Can you work these out from the model? Positions are in its coordinate system, mm. A direction names the side the tool comes from. Round coordinates to 2 decimals unless told otherwise and drop trailing zeros. Order: outer loops, then holes, each group sorted by start corner. A loop starts at its lowest first (then second) coordinate and runs counter-clockwise, first axis right, second up. Notation, with made-up numbers: (87.25, 18.5) -> (118.25, 18.5) arc R24 cw to (118.25, 28.5) -> close; hole circle Ø8 at (62.25, -13). An arc over 180 degrees is marked (long way). One line per item, written item: value.
```python
from build123d import *

# Parameters (mm, degrees)
SKETCH2_W                = 10
SKETCH2_H                = 20
BOSS_EXTRUDE1_DEPTH      = 2
BOSS_EXTRUDE1_2_DEPTH    = 2
SKETCH6_R                = 1.5
CUT_EXTRUDE1_DEPTH       = 2
BOSS_EXTRUDE2_DEPTH      = 15
BOSS_EXTRUDE2_DEPTH_BACK = 5
SKETCH7_W                = 82.998753655
SKETCH7_H                = 2
SKETCH8_R                = 1.5
SKETCH8_W                = 16
SKETCH8_H                = 2.75
CUT_EXTRUDE2_DEPTH       = 15
SKETCH9_W                = 20.030400643
SKETCH9_H                = 3
SKETCH9_W_2              = 20.007179251
CUT_EXTRUDE3_DEPTH       = 15


with BuildPart() as part:
    # Sketch2 → Boss-Extrude1 (new body)
    with BuildSketch(Plane.XY):
        with Locations((7.834645669, 10)):
            Rectangle(SKETCH2_W, SKETCH2_H)
    extrude(amount=BOSS_EXTRUDE1_DEPTH)


with BuildPart() as body_2:
    # Sketch2 → Boss-Extrude1 2 (new body)
    with BuildSketch(Plane.XY):
        with Locations((80.834645669, 10)):
            Rectangle(SKETCH2_W, SKETCH2_H)
    extrude(amount=BOSS_EXTRUDE1_2_DEPTH)


with BuildPart() as cut_extrude1_tool:
    # Sketch6 → Cut-Extrude1 (new body)
    with BuildSketch(Plane(origin=(0, 0, 0), x_dir=(-1, 0, 0), z_dir=(0, 0, -1))):
        with Locations((-80.943458849, 13)):
            Circle(SKETCH6_R)
        with Locations((-7.943458849, 13)):
            Circle(SKETCH6_R)
    extrude(amount=-CUT_EXTRUDE1_DEPTH)


with BuildPart() as part_1:
    add(part.part)

    # Cut-Extrude1: cut by cut_extrude1_tool
    add(cut_extrude1_tool.part, mode=Mode.SUBTRACT)



with BuildPart() as body_2_1:
    add(body_2.part)

    # Cut-Extrude1: cut by cut_extrude1_tool
    add(cut_extrude1_tool.part, mode=Mode.SUBTRACT)


with BuildPart() as part_2:
    add(part_1.part)

    add(body_2_1.part)  # Boss-Extrude2 merges body 2
    # Sketch7 → Boss-Extrude2 (add, two sides: drawn at the far end of the back side and taken through both)
    with BuildSketch(Plane.XY.offset(2).offset(-BOSS_EXTRUDE2_DEPTH_BACK)):
        with Locations((44.334022496, -1)):
            Rectangle(SKETCH7_W, SKETCH7_H)
    extrude(amount=BOSS_EXTRUDE2_DEPTH + BOSS_EXTRUDE2_DEPTH_BACK)

    # Sketch8 → Cut-Extrude2 (cut)
    with BuildSketch(Plane.XZ.offset(2)):
        with Locations(Location((54.084645669, 5.796272293, 0), (0, 0, 270))):
            Circle(SKETCH8_R)
        with Locations(Location((34.584645669, 5.796272293, 0), (0, 0, 270))):
            Circle(SKETCH8_R)
        with Locations((44.334645669, 1.671272293)):
            Rectangle(SKETCH8_W, SKETCH8_H)
        Polygon((24.584645669, 12.752716477), (24.584645669, 3), (2.834645669, 3), (2.834645669, 17), (85.833399324, 17), (85.833399324, 3), (64.084645669, 3), (64.084645669, 12.752716477), align=None)
    extrude(amount=-CUT_EXTRUDE2_DEPTH, mode=Mode.SUBTRACT)

    # Sketch9 → Cut-Extrude3 (cut)
    with BuildSketch(Plane(origin=(0, 0, 0), x_dir=(1, 0, 0), z_dir=(0, 1, 0))):
        with Locations((12.849845991, 1.5)):
            Rectangle(SKETCH9_W, SKETCH9_H)
        with Locations((75.829809699, 1.5)):
            Rectangle(SKETCH9_W_2, SKETCH9_H)
    extrude(amount=-CUT_EXTRUDE3_DEPTH, mode=Mode.SUBTRACT)


solid = part_2.part
```
Q1. I want a section at B-B on y = 9.5. List the corners of the cut face in (x, z) for me, plus the area to 3 significant figures.
Answers below:
outline: (2.83, 0) -> (12.83, 0) -> (12.83, 2) -> (2.83, 2) -> close; (75.83, 0) -> (85.83, 0) -> (85.83, 2) -> (75.83, 2) -> close
area: 40.0 mm^2
Q2. Please list where these lines run through material, in increasing order: line 1 along X through (y, z) = (7.75, 1); line 2 along Z through (x, y) = (12, 18.25); line 3 along Y through (x, z) = (27, 3).
Answers below:
line 1: 2.83 to 12.83, 75.83 to 85.83
line 2: 0 to 2
line 3: -2 to 0
Q3. I want a section at D-D on x = 12. List the corners of the cut face in (y, z) for me, plus the area to 3 significant figures.
Answers below:
outline: (-2, 0) -> (20, 0) -> (20, 2) -> (0, 2) -> (0, 3) -> (-2, 3) -> close
area: 46.0 mm^2
Q4. I want a section at C-C on y = 13. List the corners of the cut face in (x, z) for me.
Answers below:
outline: (2.83, 0) -> (6.44, 0) -> (6.44, 2) -> (2.83, 2) -> close; (9.44, 0) -> (12.83, 0) -> (12.83, 2) -> (9.44, 2) -> close; (75.83, 0) -> (79.44, 0) -> (79.44, 2) -> (75.83, 2) -> close; (82.44, 0) -> (85.83, 0) -> (85.83, 2) -> (82.44, 2) -> close
Q5. Will these pins go through, and if not, where does the flat tip stop? pin 1 Ø0.6 at (y, z) = (-1, -1.5) entering from +X; pin 2 Ø5 at (x, z) = (54.08, 5.8) entering from -Y; pin 3 Ø2 at (x, z) = (69.5, 0) entering from +Y; pin 4 Ø0.6 at (y, z) = (-1.5, 8.5) entering from -X.
Answers below:
pin 1: x = 65.83
pin 2: y = -2
pin 3: y = 0
pin 4: x = 24.58
Q6. I want a section at A-A on x = 51. List the corners of the cut face in (y, z) for me, plus the area to 3 significant figures.
Answers below:
outline: (-2, -3) -> (0, -3) -> (0, 0.3) -> (-2, 0.3) -> close; (-2, 3.05) -> (0, 3.05) -> (0, 12.75) -> (-2, 12.75) -> close
area: 26.0 mm^2
Q7. We'd pull the mould along X, two halves only. Please class faces 5 (the face through (65.826, -1, -1)), 6 (the face through (36.335, -1, 2)), 7 (the face through (75, -1, 3)), 8 (the face through (12.835, 10, 1)): released by +X, released by -X, zero draft, split by the parting line, or undercut.
Answers below:
face 5: released by +X
face 6: undercut
face 7: zero draft
face 8: undercut
Q8. On a 3-axis mill with a long thin cutter (end or side, diameter ignored), from which of +Z, -Z, +X, -X, +Y, -Y can I reach the whole of each face in a straight line? I mean faces 1 (the face through (24.585, -1, 8)), 2 (the face through (80, 7, 0)), 3 (the face through (8, 9, 0)), 4 (the face through (44, -1, 0.296)). Say none if no direction works.
Answers below:
face 1: +Z, -X, +Y, -Y
face 2: -Z, +X, +Y, -Y
face 3: -Z, -X, +Y, -Y
face 4: +Y, -Y
